Work out the finished part from the listing and answer in its coordinate system (mm). Coordinates: 2 decimals unless noted, no trailing zeros.
```python
from build123d import *

# Parameters (mm, degrees)
SKETCH1_W           = 150
SKETCH1_H           = 20
BOSS_EXTRUDE1_DEPTH = 10
CUT_EXTRUDE1_START  = -10
CUT_EXTRUDE1_DEPTH  = 20


# Read off the part's stored shape, not the designer's step: Cut-Extrude1
with BuildPart() as part:
    # Sketch1 → Boss-Extrude1 (new body)
    with BuildSketch(Plane(origin=(0, 0, 0), x_dir=(1, 0, 0), z_dir=(0, 1, 0))):
        with Locations((75, 0)):
            Rectangle(SKETCH1_W, SKETCH1_H)
    extrude(amount=BOSS_EXTRUDE1_DEPTH)

    # Cut-Extrude1 outline → Cut-Extrude1 (cut)
    with BuildSketch(Plane.XY.offset(CUT_EXTRUDE1_START)):
        with BuildLine():
            Line((145.663706144, 10), (82.885627876, 10))
            add(Edge.make_bspline(
                [(82.885627876, 10), (83.454977242, 9.99908028), (85.189856894, 9.956715888), (87.907695594, 9.701054679), (91.559145724, 8.993968627), (95.686256106, 7.87353082), (99.738781969, 6.629157705), (103.976290755, 5.384778121), (108.462250932, 4.377105952), (113.07700456, 3.880999352), (117.435005853, 4.040590194), (121.419605992, 4.675271787), (124.770171836, 5.486196921), (127.524123563, 6.268788566), (130.011090761, 7.016713264), (132.243780847, 7.687596399), (134.256371731, 8.261450185), (136.051140973, 8.727311429), (137.62554634, 9.089746646), (138.975122408, 9.362602964), (140.280663194, 9.584826082), (141.395781757, 9.73738392), (142.317885087, 9.837112449), (143.042775212, 9.899645746), (143.62744465, 9.939940775), (144.131855587, 9.966526877), (144.563142562, 9.98303354), (144.948720651, 9.992572398), (145.266405122, 9.997664685), (145.481284706, 9.999575397), (145.602944701, 10), (145.663706144, 10)],
                knots=[0.500349192, 0.500349192, 0.500349192, 0.500349192, 0.500349192, 0.515137701, 0.545413215, 0.571111647, 0.596810078, 0.626167806, 0.655525534, 0.685801031, 0.716076475, 0.746351906, 0.768391073, 0.790430241, 0.805568, 0.82070576, 0.83584352, 0.850981279, 0.859920909, 0.868860539, 0.877800169, 0.886739799, 0.894308658, 0.898093088, 0.901877518, 0.905661948, 0.909446378, 0.911338593, 0.913230808, 0.915123023, 0.917015238, 0.917015238, 0.917015238, 0.917015238, 0.917015238], degree=4))
        make_face()
        with BuildLine():
            add(Edge.make_bspline(
                [(20, 10), (20.060761442, 10), (20.182421455, 9.999575397), (20.39730103, 9.997664685), (20.714985555, 9.992572396), (21.100563711, 9.983033535), (21.531850968, 9.966526863), (22.036257221, 9.939940915), (22.620943851, 9.899645334), (23.345787497, 9.837113466), (24.096799885, 9.755896382), (24.871456236, 9.654807845), (25.840152712, 9.50702943), (26.68771304, 9.358248058), (27.532076328, 9.192071608), (28.373135333, 9.010270215), (29.044068, 8.856194438), (30.112337945, 8.597574089), (31.5728561, 8.214295395), (33.419910315, 7.687526736), (35.652632055, 7.016810348), (37.733272252, 6.390851426), (39.669106538, 5.834266358), (41.872853105, 5.249081541), (44.663768524, 4.608489653), (48.228694342, 4.040548399), (52.586705214, 3.881024842), (57.20145294, 4.377090051), (61.687417049, 5.384789657), (65.924923136, 6.629150647), (69.977450635, 7.873534607), (74.104560079, 8.993966893), (77.756009619, 9.701054871), (80.473847019, 9.956715992), (82.208725521, 9.999080282), (82.77807377, 10)],
                knots=[0.082984762, 0.082984762, 0.082984762, 0.082984762, 0.082984762, 0.084876977, 0.086769192, 0.088661407, 0.090553622, 0.094338052, 0.098122482, 0.101906912, 0.105691342, 0.113260201, 0.117730016, 0.122199831, 0.131139461, 0.135609276, 0.140079091, 0.144548906, 0.149018721, 0.16415648, 0.17929424, 0.194432, 0.209569759, 0.220589343, 0.231608927, 0.253648094, 0.283923525, 0.314198969, 0.344474466, 0.373832194, 0.403189922, 0.428888353, 0.454586785, 0.484862299, 0.499650779, 0.499650779, 0.499650779, 0.499650779, 0.499650779], degree=4))
            Line((82.77807377, 10), (20, 10))
        make_face()
    extrude(amount=CUT_EXTRUDE1_DEPTH, mode=Mode.SUBTRACT)


solid = part.part
```
1. Straight lines are drawn through the part: probe 1 along Y at (x, z) = (117.5, -6); probe 2 along Y at (x, z) = (76.5, -8.25). For each, find the intervals that lie inside material, in ascending order.
2. A cutting plane is placed at A-A, the plane y = 8.75. Count the separate pieces of the cut face and the enclosed holes in it, then the cut area to 3 significant figures.
3. This flat-tipped pin is pushed along its axis until it touches: P1, Ø1.5, axis at x = 17.5, z = 1.5, coming from the -Y side. Where does it stop, or does it pass through?
Answers below:
1. probe 1: y = 0 to 4.16
1. probe 2: y = 0 to 9.42
2. separate pieces: 3
2. enclosed holes: 0
2. area: 1,250 mm2
3. P1: stops at y = 0
